Autodesk Fusion 360 part; units mm, degrees
sketch "Sketch1" plane through (0, 0, 0) normal (0, 1, 0) x (1, 0, 0)
  line L0 (0, 0) -> (180, 0)
  line L1 (180, 0) -> (180, 70)
  line L2 (180, 70) -> (0, 70)
  line L3 (0, 70) -> (0, 0)
  dimension "d1" = 180
  dimension "d2" = 70
extrude "Extrude1" add sketch "Sketch1" along normal blind 5
sketch "Sketch2" plane through (0, 0, 0) normal (-1, 0, 0) x (0, 0, 1)
  line L0 (-70, 0) -> (0, 0)
  line L1 (0, 0) -> (0, 5)
  line L2 (0, 5) -> (-70, 5)
  line L3 (-70, 5) -> (-70, 0)
  line L4 (-70, 5) -> (-70, 105) construction
  line L5 (0, 5) -> (-70, 75)
  line L6 (-9.8995, 5) -> (-70, 65.1005)
  line L7 (-70, 65.1005) -> (-60.1005, 65.1005)
  line L8 (-9.8995, 5) -> (0, 5)
  dimension "d5" = 100
  dimension "d6" = 45
extrude "Extrude2" add sketch "Sketch2" against normal blind 5 contours L2 L5 L6 L7 L8
ref_plane "WorkPlane1" through (2.5, 65.1005, -70) normal (0, -0.7071, 0.7071) x (1, 0, 0)
sketch "Sketch3" plane through (0, 67.5503, -67.5503) normal (0, -0.7071, 0.7071) x (1, 0, 0)
  line L0 (0, -3.4645) -> (0, 3.5355) construction
  line L1 (0, 3.5355) -> (5, 3.5355) construction
  line L2 (5, 3.5355) -> (5, -3.4645) construction
  line L3 (5, -3.4645) -> (0, -3.4645) construction
  line L4 (5, 1.1355) -> (2.2, 1.1355)
  line L5 (2.2, 1.1355) -> (2.2, -1.0645)
  line L6 (2.2, -1.0645) -> (5, -1.0645)
  line L7 (5, -1.0645) -> (5, 1.1355)
  line L8 (5, 0.0355) -> (5, 3.5355)
  line L9 (5, 0.0355) -> (5, -3.4645)
  dimension "d11" = 2.8
  dimension "d12" = 2.2
extrude "Extrude3" cut sketch "Sketch3" along normal up to surface end surface through (0, 5, 0) normal (0, 1, 0) offset 0
sketch "Sketch4" plane through (0, 5, 0) normal (0, 1, 0) x (-1, 0, 0)
  line L0 (0, -9.8995) -> (-5, -9.8995)
  line L1 (-5, -9.8995) -> (-5, -6.5054)
  line L2 (-5, -6.5054) -> (-2.2, -6.5054)
  line L3 (-2.2, -6.5054) -> (-2.2, -3.3941)
  line L4 (-2.2, -3.3941) -> (-5, -3.3941)
  line L5 (-5, -3.3941) -> (-5, 0)
  line L6 (-5, 0) -> (-180, 0)
  line L7 (-180, 0) -> (-180, -70)
  line L8 (-180, -70) -> (0, -70)
  line L9 (0, -70) -> (0, -9.8995)
  line L10 (-2.2, -66.6059) -> (-5, -66.6059)
  line L11 (-5, -66.6059) -> (-5, -70)
  line L12 (-5, -70) -> (0, -70)
  line L13 (0, -70) -> (0, -60.1005)
  line L14 (0, -60.1005) -> (-5, -60.1005)
  line L15 (-5, -60.1005) -> (-5, -63.4946)
  line L16 (-5, -63.4946) -> (-2.2, -63.4946)
  line L17 (-2.2, -63.4946) -> (-2.2, -66.6059)
  line L18 (-5, -66.6059) -> (-2.2, -66.6059)
  line L19 (-2.2, -66.6059) -> (-2.2, -6.5054)
  line L20 (-2.2, -6.5054) -> (-5, -6.5054)
  line L21 (-5, -6.5054) -> (-5, -66.6059)
  line L22 (-5, -60.1005) -> (0, -60.1005)
  line L23 (0, -60.1005) -> (0, -70)
  line L24 (0, -70) -> (-5, -70)
  line L25 (-5, -70) -> (-5, -60.1005)
  line L26 (-5, -40.1005) -> (0, -40.1005)
  line L27 (-5, -50) -> (-5, -40.1005)
  line L28 (0, -40.1005) -> (0, -50)
  line L29 (0, -50) -> (-5, -50)
  line L30 (-5, -20.1005) -> (0, -20.1005)
  line L31 (-5, -30) -> (-5, -20.1005)
  line L32 (0, -20.1005) -> (0, -30)
  line L33 (0, -30) -> (-5, -30)
  dimension "d19" = 20
  dimension "d20" = 0
extrude "Extrude4" add sketch "Sketch4" along normal up to surface contours L9 L19 L30 L32 L33 | L19 L21 L30 L31 L33 | L9 L19 L26 L28 L29 | L19 L21 L26 L27 L29 | L8 L9 L10 L11 L12 L13 L14 L17 L18 L19 L22 L23 L24 L25 | L14 L15 L16 L19 L21 L22 L25 | L10 L16 L17 L18 L19 L21 L25 end surface through (0, 5, -9.8995) normal (0, -0.707107, -0.707107) offset 0
ref_plane "WorkPlane2" through (90, 32.5503, -35) normal (-1, 0, 0) x (0, 0, 1)
mirror "Mirror1" about plane through (90, 32.5503, -35) normal (-1, 0, 0) of "Extrude2", "Extrude4", "Extrude3"
sketch "Sketch5" plane through (0, 0, 0) normal (0, -1, 0) x (1, 0, 0)
  line L0 (0, 0) -> (0, -70)
  line L1 (0, -70) -> (180, -70)
  line L2 (180, -70) -> (180, 0)
  line L3 (180, 0) -> (0, 0)
  line L4 (180, -35) -> (0, -35) construction
  line L5 (90, -70) -> (90, 0) construction
  circle A0 centre (140, -35) radius 15.5
  circle A1 centre (40, -35) radius 15.5
  dimension "d23" = 31
  dimension "d24" = 50
extrude "Extrude5" cut sketch "Sketch5" against normal blind 2.5 contours A0 | A1
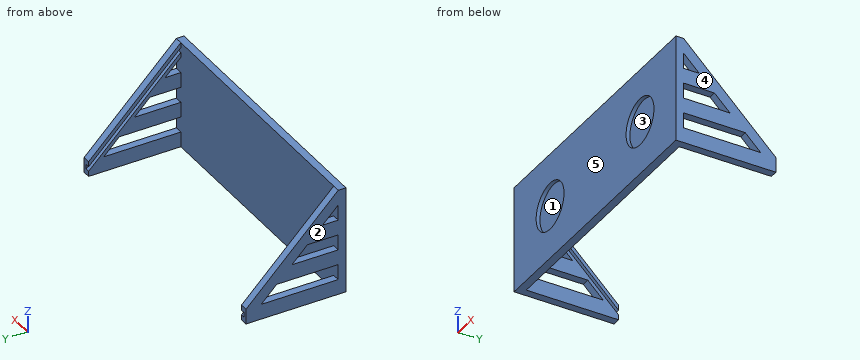
Can you work these out from the model? Positions are in its coordinate system, mm. Face numbers are marked on the shaded views. A direction names the side the tool comes from. Round coordinates to 2 decimals unless told otherwise and drop trailing zeros. Loops run counter-clockwise (first coordinate to the right, second up) from the corner with the lowest first, then second, coordinate; pieces in that order, holes last.
Item 1: Suppose I cut it at C-C, the plane x = 40. Write out the boundary of the cut face in (y, z).
Item 2: Please list where these lines run through material, in increasing order: L1, parallel to Z at x = 140, y = 1; L2, parallel to X at y = 27.5, z = -27; L3, parallel to Y at x = 102, z = -31.5.
Item 3: If we mould it in two halves opening along X, with no side actions, what happens to the marked faces 3, 4 and 5? For each: +X half, -X half, draft (parallel to the pull), parting line (faces both ways), or undercut.
Item 4: Will these pins go through, and if not, where does the flat tip stop? pin 1 Ø15.5 at (x, z) = (133, -37.5) entering from -Y; pin 2 Ø1.5 at (x, y) = (3.5, 11) entering from +Z; pin 3 Ø10 at (x, z) = (131.5, -52) entering from -Y; pin 4 Ø5.5 at (x, y) = (2, 21.5) entering from +Z.
Item 5: Which directions (+Z, -Z, +X, -X, +Y, -Y) give clear straight access to the entire face, cutting with the end or side of a thin tool? Please do the marked faces 1 and 2.
Item 6: Suppose I cut it at A-A, the plane z = -35. Write out the boundary of the cut face in (x, y).
Item 7: Suppose I cut it at B-B, the plane y = 29. State how many separate pieces and enclosed holes the cut face has, then the cut area to 3 significant figures.
Item 8: Suppose I cut it at D-D, the plane z = -46. Write out the boundary of the cut face in (x, y).
Reported:
1. outline: (0, -70) - (5, -70) - (5, 0) - (0, 0) - (0, -19.5) - (2.5, -19.5) - (2.5, -50.5) - (0, -50.5) - close
2. L1: z = -70 to -50.5, -19.5 to 0
2. L2: x = 0 to 2.2, 177.8 to 180
2. L3: y = 0 to 5
3. face 3: undercut
3. face 4: +X half
3. face 5: draft
4. pin 1: stops at y = 2.5
4. pin 2: stops at z = -5.25
4. pin 3: stops at y = 0
4. pin 4: stops at z = -13.75
5. face 1: -Y
5. face 2: +Z, -Z, -X, +Y, -Y
6. outline: (0, 0) - (24.5, 0) - (24.5, 2.5) - (55.5, 2.5) - (55.5, 0) - (124.5, 0) - (124.5, 2.5) - (155.5, 2.5) - (155.5, 0) - (180, 0) - (180, 5) - (0, 5) - close; (0, 30.1) - (5, 30.1) - (5, 33.49) - (2.2, 33.49) - (2.2, 36.61) - (5, 36.61) - (5, 40) - (0, 40) - close; (175, 30.1) - (180, 30.1) - (180, 40) - (175, 40) - (175, 36.61) - (177.8, 36.61) - (177.8, 33.49) - (175, 33.49) - close
7. separate pieces: 6
7. enclosed holes: 0
7. area: 280 mm2
8. outline: (0, 0) - (29.08, 0) - (29.08, 2.5) - (50.92, 2.5) - (50.92, 0) - (129.08, 0) - (129.08, 2.5) - (150.92, 2.5) - (150.92, 0) - (180, 0) - (180, 51) - (175, 51) - (175, 47.61) - (177.8, 47.61) - (177.8, 44.49) - (175, 44.49) - (175, 5) - (5, 5) - (5, 44.49) - (2.2, 44.49) - (2.2, 47.61) - (5, 47.61) - (5, 51) - (0, 51) - close
